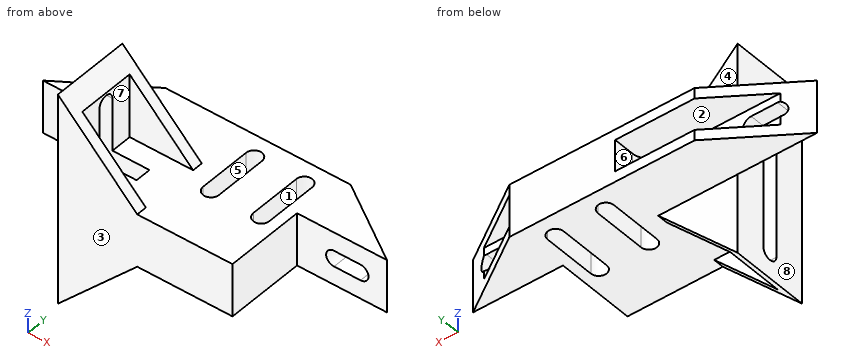
from build123d import *

# Parameters (mm, degrees)
PAD015_DEPTH    = 10
PAD016_DEPTH    = 15
SKETCH104_W     = 17.509207
SKETCH104_H     = 6
SKETCH104_W_2   = 32.035683
POCKET034_DEPTH = 7
POCKET035_DEPTH = 5
FILLET011_R     = 3
SKETCH106_W     = 11
SKETCH106_H     = 13
POCKET036_DEPTH = 32
POCKET037_DEPTH = 10
SKETCH108_W     = 15
SKETCH108_H     = 10
POCKET038_DEPTH = 2


with BuildPart() as part:
    # Sketch102 → Pad015 (new body)
    with BuildSketch(Plane.XY):
        Polygon((0, 0), (0, 15), (15, 15), (0, 25), (-35, 25), (-50, 15), (-35, 15), (-35, 0), align=None)
        with BuildLine():
            ThreePointArc((-4, 21), (-5.5, 22.5), (-7, 21))
            Line((-7, 21), (-7, 11))
            ThreePointArc((-7, 11), (-5.5, 9.5), (-4, 11))
            Line((-4, 21), (-4, 11))
        make_face(mode=Mode.SUBTRACT)
        with BuildLine():
            ThreePointArc((-13.5, 21), (-15, 22.5), (-16.5, 21))
            Line((-16.5, 21), (-16.5, 11))
            ThreePointArc((-16.5, 11), (-15, 9.5), (-13.5, 11))
            Line((-13.5, 21), (-13.5, 11))
        make_face(mode=Mode.SUBTRACT)
    extrude(amount=PAD015_DEPTH)

    # Sketch103 (on Face2 of Pad015) → Pad016 (join)
    with BuildSketch(Plane.XZ):
        Polygon((-35, 10), (-35, 25), (-20, 10), align=None)
        Polygon((-20, 0), (-35, 0), (-35, -15), align=None)
    extrude(amount=-PAD016_DEPTH)

    # Sketch104 (on Face10 of Pad016) → Pocket034 (cut)
    with BuildSketch(Plane(origin=(0, 25, 0), x_dir=(-1, 0, 0), z_dir=(0, 1, 0))):
        with Locations((-8.754603, 5)):
            Rectangle(SKETCH104_W, SKETCH104_H)
        with Locations((36.017842, 5)):
            Rectangle(SKETCH104_W_2, SKETCH104_H)
    extrude(amount=-POCKET034_DEPTH, mode=Mode.SUBTRACT)

    # Sketch105 (on Face1 of Pocket034) → Pocket035 (cut)
    with BuildSketch(Plane.XZ.offset(-15)):
        with BuildLine():
            ThreePointArc((10, 3.5), (11.5, 5), (10, 6.5))
            Line((10, 6.5), (5, 6.5))
            ThreePointArc((5, 6.5), (3.5, 5), (5, 3.5))
            Line((10, 3.5), (5, 3.5))
        make_face()
        with BuildLine():
            ThreePointArc((-45, 6.5), (-46.5, 5), (-45, 3.5))
            Line((-45, 3.5), (-40, 3.5))
            ThreePointArc((-40, 3.5), (-38.5, 5), (-40, 6.5))
            Line((-45, 6.5), (-40, 6.5))
        make_face()
    extrude(amount=-POCKET035_DEPTH, mode=Mode.SUBTRACT)

    # Fillet011
    fillet011_edges = [part.edges().sort_by_distance(p)[0] for p in [
        (-20, 18, 5),
        (0, 18, 5),
    ]]
    fillet(fillet011_edges, radius=FILLET011_R)

    # Sketch106 (on Face18 of Fillet011) → Pocket036 (cut)
    with BuildSketch(Plane.YZ):
        with Locations((7.5, 16.5)):
            Rectangle(SKETCH106_W, SKETCH106_H)
        with Locations((7.5, -6.5)):
            Rectangle(SKETCH106_W, SKETCH106_H)
    extrude(amount=-POCKET036_DEPTH, mode=Mode.SUBTRACT)

    # Sketch107 (on Face17 of Pocket036) → Pocket037 (cut)
    with BuildSketch(Plane(origin=(-35, 0, 0), x_dir=(0, -1, 0), z_dir=(-1, 0, 0))):
        with BuildLine():
            ThreePointArc((-6, 20), (-7.5, 21.5), (-9, 20))
            Line((-9, 20), (-9, -10))
            ThreePointArc((-9, -10), (-7.5, -11.5), (-6, -10))
            Line((-6, 20), (-6, -10))
        make_face()
    extrude(amount=-POCKET037_DEPTH, mode=Mode.SUBTRACT)

    # Sketch108 (on Face26 of Pocket037) → Pocket038 (cut)
    with BuildSketch(Plane.YZ):
        with Locations((7.5, 5)):
            Rectangle(SKETCH108_W, SKETCH108_H)
    extrude(amount=-POCKET038_DEPTH, mode=Mode.SUBTRACT)


with BuildPart() as part_1:
    # Body008 placement: moved
    add(part.part.moved(Location((-38, -112, 32))))


solid = part_1.part
Part model, mm, in its own coordinate system. Face numbers are marked on the shaded views. A direction names the side the tool comes from. Give positions to 0.01 mm unless a question says otherwise; leave off trailing zeros. Order: outer loops, then holes, each group sorted by start corner. A loop starts at its lowest first (then second) coordinate and runs counter-clockwise, first axis right, second up. Notation, with made-up numbers: (-6, 45) - (34, 45) arc R24 cw to (34, 81) - close; hole circle Ø5 at (-22, 30). An arc over 180 degrees is marked (long way). One line per question, with ' | ' between items.
1. Which spindle directions (+Z, -Z, +X, -X, +Y, -Y) get a long thin tool onto all of the face, cutting with end or side? Do the marked faces 4, 5, 6, 7 and 8. Say none if no direction does.
Filled in:
face 4: +Z, +X, -X, +Y | face 5: +Z, -Z | face 6: -X, +Y | face 7: +Z, +X | face 8: +Z, -Z, -X, -Y
2. Pull direction Y, two halves, no side cores. Call the marked faces 1, 2 and 3: +Y half, -Y half, draft (parallel to the pull), parting line (faces both ways), or undercut.
Filled in:
face 1: undercut | face 2: draft | face 3: -Y half
3. Band-saw the part on B-B on y = -104.5. List the corners of the cut face in (x, z), then the cut area to 3 significant figures.
Filled in:
outline: (-73, 17) - (-70, 20) - (-70, 20.5) - (-73, 20.5) - close; (-73, 53.5) - (-70, 53.5) - (-70, 54) - (-73, 57) - close; (-63, 32) - (-40, 32) - (-40, 42) - (-63, 42) - close | area: 242 mm²
4. Band-saw the part on C-C on x = -65. List the corners of the cut face in (y, z).
Filled in:
outline: (-112, 25) - (-110, 25) - (-110, 32) - (-106, 32) - (-106, 42) - (-110, 42) - (-110, 49) - (-112, 49) - close; (-103, 32) - (-99, 32) - (-99, 25) - (-97, 25) - (-97, 32) - (-87, 32) - (-87, 34) - (-94, 34) - (-94, 40) - (-87, 40) - (-87, 42) - (-97, 42) - (-97, 49) - (-99, 49) - (-99, 42) - (-103, 42) - close
5. Drill centre lines: probe 1 along X at (y, z) = (-91, 35.5); probe 2 along Z at (x, y) = (-81, -93.5); probe 3 along Y at (x, z) = (-72.5, 47.5). Where is each one in solid material? Low to high.
Filled in:
probe 1: -58 to -54.5, -51.5 to -45, -42 to -38 | probe 2: 32 to 34, 40 to 42 | probe 3: -112 to -106, -103 to -97
6. Band-saw the part on D-D on z = 37. Give the number of separate pieces and of enclosed holes in the cut face, then the cut area to 3 significant figures.
Filled in:
separate pieces: 3 | enclosed holes: 2 | area: 669 mm²
7. Drop flat-ended pins along their axis: P1, Ø12, axis at y = -105.5, z = 23.5, coming from the +X side; P2, Ø10, axis at x = -63.5, y = -90.5, coming from the +Z side; P3, Ø6, axis at y = -106, z = 45.5, coming from the -X side. Give the stop position or say it passes through.
Filled in:
P1: x = -62.53 | P2: z = 42 | P3: x = -73
8. Band-saw the part on A-A on z = 30. List the corners of the cut face in (x, y), then the cut area to 3 significant figures.
Filled in:
outline: (-73, -112) - (-60, -112) - (-60, -110) - (-70, -110) - (-70, -106) - (-73, -106) - close; (-73, -103) - (-70, -103) - (-70, -99) - (-60, -99) - (-60, -97) - (-73, -97) - close | area: 76.0 mm²
